from build123d import *

# Parameters (mm, degrees)
F0_W     = 25
F0_H     = 30
F1_DEPTH = 2
F2_R     = 1.5
F3_DEPTH = 2.001
F4_W     = 25
F4_H     = 6.1
F5_DEPTH = 0.9
F6_SIZE  = 10
F7_R     = 7


with BuildPart() as f1:
    # F0 (on Top) → F1 (new body)
    with BuildSketch(Plane.XY):
        Rectangle(F0_W, F0_H)
    extrude(amount=F1_DEPTH)

    # F2 (on face) → F3 (cut, through all)
    with BuildSketch(Plane.XY.offset(2)):
        with Locations((-2, -12)):
            Circle(F2_R)
        with Locations((4.5, -1.5)):
            Circle(F2_R)
        with Locations((4.5, 8.5)):
            Circle(F2_R)
    extrude(amount=-F3_DEPTH, mode=Mode.SUBTRACT)

    # F4 (on face) → F5 (cut)
    with BuildSketch(Plane(origin=(0, 0, 0), x_dir=(1, 0, 0), z_dir=(0, 0, -1))):
        with Locations((0, -3.051)):
            Rectangle(F4_W, F4_H)
    extrude(amount=-F5_DEPTH, mode=Mode.SUBTRACT)

    # F6
    f6_edges = [f1.edges().sort_by_distance(p)[0] for p in [
        (-12.5, 15, 1),
    ]]
    chamfer(f6_edges, length=F6_SIZE)

    # F7
    f7_edges = [f1.edges().sort_by_distance(p)[0] for p in [
        (-12.5, 5, 1.45),
        (-2.5, 15, 1),
        (12.5, 15, 1),
    ]]
    fillet(f7_edges, radius=F7_R)


solid = f1.part
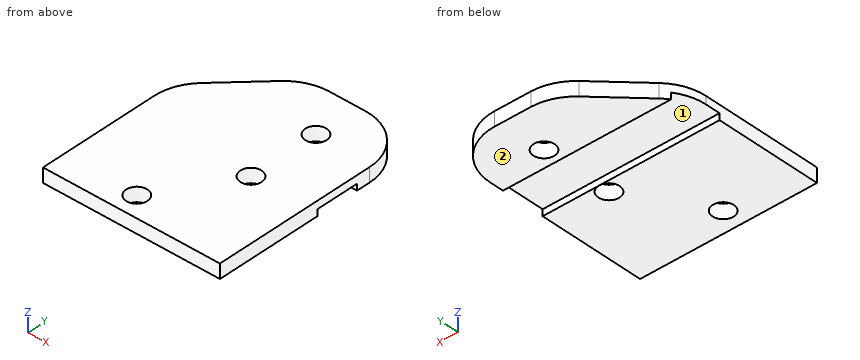
Work out the finished part from the listing and answer in its coordinate system (mm). Face numbers are marked on the shaded views. Round coordinates to 2 decimals unless told otherwise and drop trailing zeros. Loops run counter-clockwise (first coordinate to the right, second up) from the corner with the lowest first, then second, coordinate; pieces in that order, holes last. Notation, with made-up numbers: (27, 28.5) - (42, 28.5) arc R26 cw to (42, 49.5) - close; hole circle Ø1 at (-20, 13). An arc over 180 degrees is marked (long way). Use one line per item in the form item = value. Start each with the question number.
(1) Find section A-A on z = 0.45. Determine the outline of the cut face in (x, y).
(2) Flat-ended cylindrical pins translate along their axes: P1, Ø3, axis at x = -2, y = 4, coming from the -Z side; P2, Ø3, axis at x = 1, y = 10, coming from the -Z side; P3, Ø1, axis at y = 6, z = 1.5, coming from the -X side. Find the tip coordinate at first contact, or state that the pin passes through.
(3) Find section B-B on y = -12. Determine the outline of the cut face in (x, z), and give its area (3 significant figures).
(4) Consider line 1 (Y direction, x = 4.5, z = 1.15); line 2 (Y direction, x = 1.5, z = 0.75); line 3 (Z direction, x = 9.75, y = 2). Determine where each line is inside the solid, lowest interval first.
(5) Find section D-D on x = -8. Determine the outline of the cut face in (y, z), and give its area (3 significant figures).
(6) Determine the mould class of the marked faces 1 and 2 for opening direction Y: +Y half, -Y half, draft (parallel to the pull), parting line (faces both ways), or undercut.
(7) Find section C-C on x = 5. Determine the outline of the cut face in (y, z).
Answer list:
q1.outline = (-12.5, -15) - (12.5, -15) - (12.5, 0) - (-12.5, 0) - close; (-11.24, 6.1) - (12.5, 6.1) - (12.5, 8) arc R7 ccw to (5.5, 15) - (0.4, 15) arc R7 ccw to (-4.55, 12.95) - (-10.45, 7.05) arc R7 ccw to start; hole circle Ø3 at (-2, -12); hole circle Ø3 at (4.5, -1.5); hole circle Ø3 at (4.5, 8.5)
q2.P1 = 0.9
q2.P2 = 0
q2.P3 = -11.62
q3.outline = (-12.5, 0) - (-3.5, 0) - (-3.5, 2) - (-12.5, 2) - close; (-0.5, 0) - (12.5, 0) - (12.5, 2) - (-0.5, 2) - close
q3.area = 44.0 mm^2
q4.line_1 = -15 to -3, 0 to 7, 10 to 15
q4.line_2 = -15 to 0, 6.1 to 15
q4.line_3 = 0.9 to 2
q5.outline = (-15, 0) - (0, 0) - (0, 0.9) - (6.1, 0.9) - (6.1, 0) - (9.5, 0) - (9.5, 2) - (-15, 2) - close
q5.area = 43.5 mm^2
q6.face_1 = undercut
q6.face_2 = draft
q7.outline = (-15, 0) - (-2.91, 0) - (-2.91, 2) - (-15, 2) - close; (-0.09, 0) - (0, 0) - (0, 0.9) - (6.1, 0.9) - (6.1, 0) - (7.09, 0) - (7.09, 2) - (-0.09, 2) - close; (9.91, 0) - (15, 0) - (15, 2) - (9.91, 2) - close
